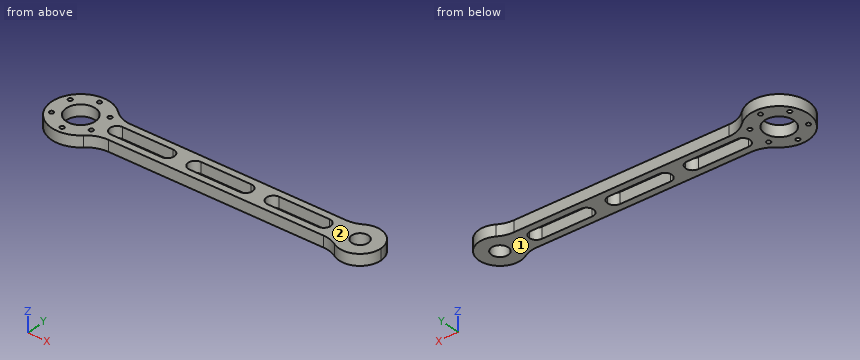
```python
from build123d import *

# Parameters (mm, degrees)
EXTRUDE_1_DEPTH     = 8
FILLET_1_R          = 20
SKETCH_5_R          = 10.5
SKETCH_5_R_2        = 6
CUT_EXTRUDE_4_DEPTH = 10
CUT_EXTRUDE_5_DEPTH = 10
EXTRUDE_START       = -8
SKETCH_9_R          = 10.5
EXTRUDE_3_DEPTH     = 8
FILLET_2_R          = 20
SKETCH_10_R         = 1.5
CUT_EXTRUDE_7_DEPTH = 8


with BuildPart() as part:
    # 草图1 → 凸台-拉伸1 (new body)
    with BuildSketch(Plane.XY):
        with BuildLine():
            Line((0, -10), (0, 10))
            Line((0, 10), (11.180339887, 10))
            ThreePointArc((11.180339887, 10), (-15, 0), (11.180339887, -10))
            Line((11.180339887, -10), (0, -10))
        make_face()
        with BuildLine():
            Line((11.180339887, 10), (0, 10))
            Line((0, 10), (0, -10))
            Line((0, -10), (11.180339887, -10))
            ThreePointArc((11.180339887, -10), (14.012585384, -5.352331347), (15, 0))
            ThreePointArc((15, 0), (14.012585384, 5.352331347), (11.180339887, 10))
        make_face()
        with BuildLine():
            Line((188.819660113, 10), (11.180339887, 10))
            ThreePointArc((11.180339887, 10), (14.012585384, 5.352331347), (15, 0))
            ThreePointArc((15, 0), (14.012585384, -5.352331347), (11.180339887, -10))
            Line((11.180339887, -10), (188.819660113, -10))
            ThreePointArc((188.819660113, -10), (185, 0), (188.819660113, 10))
        make_face()
        with BuildLine():
            ThreePointArc((215, 0), (205.352331347, 14.012585384), (188.819660113, 10))
            Line((188.819660113, 10), (200, 10))
            Line((200, 10), (200, -10))
            Line((200, -10), (188.819660113, -10))
            ThreePointArc((188.819660113, -10), (205.352331347, -14.012585384), (215, 0))
        make_face()
        with BuildLine():
            Line((200, 10), (188.819660113, 10))
            ThreePointArc((188.819660113, 10), (185, 0), (188.819660113, -10))
            Line((188.819660113, -10), (200, -10))
            Line((200, -10), (200, 10))
        make_face()
    extrude(amount=EXTRUDE_1_DEPTH)

    # 圆角1
    fillet_1_edges = [part.edges().sort_by_distance(p)[0] for p in [
        (11.180339887, 10, 4),
        (188.819660113, 10, 4),
        (188.819660113, -10, 4),
        (11.180339887, -10, 4),
    ]]
    fillet(fillet_1_edges, radius=FILLET_1_R)

    # 草图5 → 切除-拉伸4 (cut)
    with BuildSketch(Plane.XY.offset(8)):
        Circle(SKETCH_5_R)
        with Locations((200, 0)):
            Circle(SKETCH_5_R_2)
    extrude(amount=-CUT_EXTRUDE_4_DEPTH, mode=Mode.SUBTRACT)

    # 草图6 → 切除-拉伸5 (cut)
    with BuildSketch(Plane.XY.offset(8)):
        with BuildLine():
            ThreePointArc((138, 5), (133, 0), (138, -5))
            Line((138, -5), (138, 5))
        make_face()
        with BuildLine():
            Line((138, 5), (138, -5))
            ThreePointArc((138, -5), (141.535533906, -3.535533906), (143, 0))
            ThreePointArc((143, 0), (141.535533906, 3.535533906), (138, 5))
        make_face()
        with BuildLine():
            Line((138, -5), (174, -5))
            ThreePointArc((174, -5), (169, 0), (174, 5))
            Line((174, 5), (138, 5))
            ThreePointArc((138, 5), (141.535533906, 3.535533906), (143, 0))
            ThreePointArc((143, 0), (141.535533906, -3.535533906), (138, -5))
        make_face()
        with BuildLine():
            ThreePointArc((174, 5), (169, 0), (174, -5))
            Line((174, -5), (174, 5))
        make_face()
        with BuildLine():
            Line((174, 5), (174, -5))
            ThreePointArc((174, -5), (177.535533906, -3.535533906), (179, 0))
            ThreePointArc((179, 0), (177.535533906, 3.535533906), (174, 5))
        make_face()
        with BuildLine():
            ThreePointArc((118, 5), (113, 0), (118, -5))
            Line((118, -5), (118, 5))
        make_face()
        with BuildLine():
            Line((118, 5), (118, -5))
            ThreePointArc((118, -5), (121.535533906, -3.535533906), (123, 0))
            ThreePointArc((123, 0), (121.535533906, 3.535533906), (118, 5))
        make_face()
        with BuildLine():
            Line((82, -5), (118, -5))
            ThreePointArc((118, -5), (113, 0), (118, 5))
            Line((118, 5), (82, 5))
            ThreePointArc((82, 5), (85.535533906, 3.535533906), (87, 0))
            ThreePointArc((87, 0), (85.535533906, -3.535533906), (82, -5))
        make_face()
        with BuildLine():
            ThreePointArc((82, 5), (77, 0), (82, -5))
            Line((82, -5), (82, 5))
        make_face()
        with BuildLine():
            Line((82, 5), (82, -5))
            ThreePointArc((82, -5), (85.535533906, -3.535533906), (87, 0))
            ThreePointArc((87, 0), (85.535533906, 3.535533906), (82, 5))
        make_face()
        with BuildLine():
            ThreePointArc((62, 5), (57, 0), (62, -5))
            Line((62, -5), (62, 5))
        make_face()
        with BuildLine():
            Line((62, 5), (62, -5))
            ThreePointArc((62, -5), (65.535533906, -3.535533906), (67, 0))
            ThreePointArc((67, 0), (65.535533906, 3.535533906), (62, 5))
        make_face()
        with BuildLine():
            Line((26, -5), (62, -5))
            ThreePointArc((62, -5), (57, 0), (62, 5))
            Line((62, 5), (26, 5))
            ThreePointArc((26, 5), (29.535533906, 3.535533906), (31, 0))
            ThreePointArc((31, 0), (29.535533906, -3.535533906), (26, -5))
        make_face()
        with BuildLine():
            ThreePointArc((26, 5), (21, 0), (26, -5))
            Line((26, -5), (26, 5))
        make_face()
        with BuildLine():
            Line((26, 5), (26, -5))
            ThreePointArc((26, -5), (29.535533906, -3.535533906), (31, 0))
            ThreePointArc((31, 0), (29.535533906, 3.535533906), (26, 5))
        make_face()
    extrude(amount=-CUT_EXTRUDE_5_DEPTH, mode=Mode.SUBTRACT)

    # 草图9 → 凸台-拉伸3 (add)
    with BuildSketch(Plane(origin=(0, 0, 0), x_dir=(-1, 0, 0), z_dir=(0, 0, -1)).offset(EXTRUDE_START)):
        with BuildLine():
            Line((-18.466185313, 10), (-18.466185313, -10))
            ThreePointArc((-18.466185313, -10), (21, 0), (-18.466185313, 10))
        make_face()
        with Locations(Location((0, 0, 0), (0, 0, 180))):
            Circle(SKETCH_9_R, mode=Mode.SUBTRACT)
    extrude(amount=EXTRUDE_3_DEPTH)

    # 圆角2
    fillet_2_edges = [part.edges().sort_by_distance(p)[0] for p in [
        (18.466185313, 10, 4),
        (18.466185313, -10, 4),
    ]]
    fillet(fillet_2_edges, radius=FILLET_2_R)

    # 草图10 → 切除-拉伸7 (cut)
    with BuildSketch(Plane(origin=(0, 0, 0), x_dir=(-1, 0, 0), z_dir=(0, 0, -1))):
        with Locations((0, 16.5)):
            Circle(SKETCH_10_R)
        with Locations((14.289419162, 8.25)):
            Circle(SKETCH_10_R)
        with Locations((14.289419162, -8.25)):
            Circle(SKETCH_10_R)
        with Locations((0, -16.5)):
            Circle(SKETCH_10_R)
        with Locations((-14.289419162, -8.25)):
            Circle(SKETCH_10_R)
        with Locations((-14.289419162, 8.25)):
            Circle(SKETCH_10_R)
    extrude(amount=-CUT_EXTRUDE_7_DEPTH, mode=Mode.SUBTRACT)


solid = part.part
```
Could you check a few things on this model? Use its own coordinates, in mm. Face numbers are marked on the shaded views. Give positions to 0.01 mm unless a question says otherwise; leave off trailing zeros. Order: outer loops, then holes, each group sorted by start corner. A loop starts at its lowest first (then second) coordinate and runs counter-clockwise, first axis right, second up.
Q1. We'd pull the mould along Z, two halves only. Please class the marked faces 1 and 2: +Z half, -Z half, draft (parallel to the pull), parting line (faces both ways), or undercut.
Q2. I'm going to push flat-ended pins straight in: P1, Ø4, axis at x = 44.5, z = 3, coming from the +Y side; P2, Ø2, axis at x = 122, y = -10.5, coming from the -Z side; P3, Ø4, axis at y = 2, z = 7, coming from the -X side; P4, Ø4, axis at x = 164, z = 6, coming from the -Y side. Where does each tip first touch, or does it pass through?
Q3. Suppose I cut it at B-B, the plane z = 3.5. Count the separate pieces of the cut face and the enclosed holes in it, and give its area (3 significant figures).
Q4. If I drill on line 1 along Y through (x, z) = (0, 2.5); line 2 along Y through (x, z) = (84, 7.5); line 3 along X through (y, z) = (4, 4.75), over which ranges is the centre line in solid material (lowest first)?
Q5. Suppose I cut it at C-C, the plane x = 200. Write out the boundary of the cut face in (y, z), and give its area (3 significant figures).
Q6. Suppose I cut it at A-A, the plane x = 50.5. Write out the boundary of the cut face in (y, z), and give its area (3 significant figures).
Solution:
1. face 1: -Z half
1. face 2: +Z half
2. P1: stops at y = 10
2. P2: stops at z = 0
2. P3: stops at x = -21
2. P4: stops at y = -10
3. separate pieces: 1
3. enclosed holes: 11
3. area: 3,620 mm2
4. line 1: y = -21 to -18, -15 to -10.5, 10.5 to 15, 18 to 21
4. line 2: y = -10 to -5, 5 to 10
4. line 3: x = -20.62 to -9.71, 9.71 to 23, 65 to 79, 121 to 135, 177 to 195.53, 204.47 to 214.46
5. outline: (-15, 0) - (-6, 0) - (-6, 8) - (-15, 8) - close; (6, 0) - (15, 0) - (15, 8) - (6, 8) - close
5. area: 144 mm2
6. outline: (-10, 0) - (-5, 0) - (-5, 8) - (-10, 8) - close; (5, 0) - (10, 0) - (10, 8) - (5, 8) - close
6. area: 80.0 mm2
